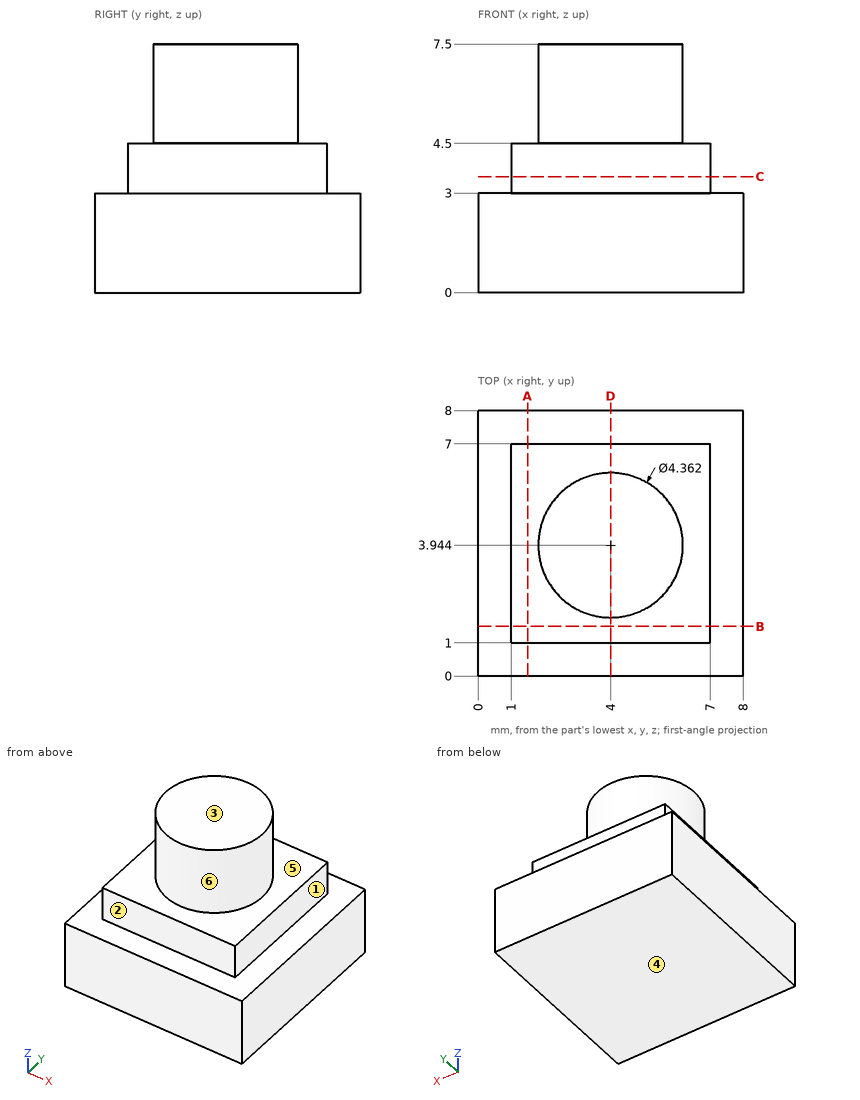
Could you check a few things on this drawing? It's one solid part, dimensions in mm from its lowest x, y, z. A direction names the side the tool comes from. Coordinates: 2 decimals unless noted, no trailing zeros. Order: outer loops, then holes, each group sorted by start corner. A loop starts at its lowest first (then second) coordinate and runs counter-clockwise, first axis right, second up. Notation, with made-up numbers: (-35.5, 79) -> (18.5, 79) arc R24 ccw to (18.5, 99) -> close; hole circle Ø2 at (89, 83). An arc over 180 degrees is marked (long way). One line per item, written item: value. Start each with the question number.
1) Which directions (+Z, -Z, +X, -X, +Y, -Y) give clear straight access to the entire face, cutting with the end or side of a thin tool? Please do the marked faces 1, 2 and 3.
2) I'm going to push flat-ended pins straight in: pin 1 (0.8 mm diameter, centred on y = 3, z = 3.5, fed in from -X); pin 2 (1.5 mm diameter, centred on x = 6.5, z = 6.5, fed in from +Y) (1 decimal); pin 3 (1.6 mm diameter, centred on y = 2.5, z = 4, fed in from +X); pin 4 (1.5 mm diameter, centred on x = 4, y = 6.5, fed in from +Z). Where does each tip first touch, or does it pass through?
3) Imagine slicing it at A-A on x = 1.5. List the corners of the cut face in (y, z) for me, plus the area to 3 significant figures.
4) If I drill on L1, parallel to Z at x = 0.5, y = 2.5; L2, parallel to Y at x = 4, z = 3.5; L3, parallel to Z at x = 6.5, y = 5.5, over which ranges is the centre line in solid material (lowest first)? Write a range as [from, to].
5) Imagine slicing it at C-C on z = 3.5. List the corners of the cut face in (x, y) for me.
6) We'd pull the mould along Z, two halves only. Please class the marked faces 4, 5 and 6: +Z half, -Z half, draft (parallel to the pull), parting line (faces both ways), or undercut.
7) Imagine slicing it at D-D on x = 4. List the corners of the cut face in (y, z) for me (1 decimal).
Answer list:
1. face 1: +Z, +X, +Y, -Y
1. face 2: +Z, +X, -X, -Y
1. face 3: +Z, +X, -X, +Y, -Y
2. pin 1: stops at x = 1
2. pin 2: stops at y = 5.2
2. pin 3: stops at x = 7
2. pin 4: stops at z = 7.5
3. outline: (0, 0) -> (8, 0) -> (8, 3) -> (7, 3) -> (7, 4.5) -> (1, 4.5) -> (1, 3) -> (0, 3) -> close
3. area: 33.0 mm2
4. L1: z = [0, 3]
4. L2: y = [1, 7]
4. L3: z = [0, 4.5]
5. outline: (1, 1) -> (7, 1) -> (7, 7) -> (1, 7) -> close
6. face 4: -Z half
6. face 5: +Z half
6. face 6: draft
7. outline: (0, 0) -> (8, 0) -> (8, 3) -> (7, 3) -> (7, 4.5) -> (6.1, 4.5) -> (6.1, 7.5) -> (1.8, 7.5) -> (1.8, 4.5) -> (1, 4.5) -> (1, 3) -> (0, 3) -> close
